CAD build for the part. Positions are in the model's coordinates, mm. A direction names the side the tool comes from. Give positions to 0.01 mm unless a question says otherwise; leave off trailing zeros. Order: outer loops, then holes, each group sorted by start corner. A loop starts at its lowest first (then second) coordinate and runs counter-clockwise, first axis right, second up.
Item 1: Wall check: L1, parallel to Y at x = 4.75, z = 13. Give the ranges that are in metal, low to high.
Item 2: Band-saw the part on C-C on z = 5. Give the cut face in (x, y).
Item 3: Band-saw the part on D-D on x = 4.05. Give the cut face in (y, z), plus the area to 3 significant figures.
Item 4: Which spindle directions (+Z, -Z, +X, -X, +Y, -Y) get a long thin tool onto all of the face, cutting with end or side? Do faces 1 (the flat face through (6.46, -2, 5)), 2 (the cylindrical face through (4.293, -0.986, 0.64)), 3 (the flat face through (0.54, -2, 5)), 4 (the flat face through (1.04, -2, 5)), 5 (the flat face through (5.96, -2, 8)). Say none if no direction does.
Item 5: Band-saw the part on B-B on x = 6.21. Give the cut face in (y, z), plus the area to 3 significant figures.
Item 6: Band-saw the part on A-A on y = -1.5. Give the cut face in (x, z).
Item 7: Two-plate mould, pull along X, no slides. Class faces 6 (the flat face through (4, 7, 13.7)), 7 (the flat face through (0, 7, 7)), 8 (the cylindrical face through (5.84, -0.99, 0.87)): released by +X, released by -X, zero draft, split by the parting line, or undercut.
Item 8: Flat gauge pins, fed straight in: P1, Ø1.2, axis at y = -1.5, z = 5.5, coming from the +X side; P2, Ø5, axis at y = -0.5, z = 3, coming from the +X side; P3, Ø1.6, axis at y = -2, z = 8, coming from the -X side; P4, Ø0.6, axis at x = 4, z = 1, coming from the -Y side. Where does each tip first touch, or does it go through?
```python
from build123d import *

# Parameters (mm, degrees)
ESQUISSE1_W      = 7.25
ESQUISSE1_H      = 14.75
EXTRUSION1_DEPTH = 13.7
EXTRUSION2_DEPTH = 3.65
ESQUISSE3_R      = 0.4
EXTRUSION3_DEPTH = 2


with BuildPart() as part:
    # Esquisse1 → Extrusion1 (new body)
    with BuildSketch(Plane.XY):
        with Locations((3.625, 7.375)):
            Rectangle(ESQUISSE1_W, ESQUISSE1_H)
    extrude(amount=EXTRUSION1_DEPTH)

    # Esquisse2 → Extrusion2 (add)
    with BuildSketch(Plane.XZ):
        with BuildLine():
            Line((1.04, 6.84), (1.04, 8.34))
            ThreePointArc((1.04, 8.34), (0.79, 8.59), (0.54, 8.34))
            Line((0.54, 8.34), (0.54, 6.84))
            ThreePointArc((0.54, 6.84), (0.79, 6.59), (1.04, 6.84))
        make_face()
        with BuildLine():
            Line((6.46, 6.84), (6.46, 8.34))
            ThreePointArc((6.46, 8.34), (6.21, 8.59), (5.96, 8.34))
            Line((5.96, 8.34), (5.96, 6.84))
            ThreePointArc((5.96, 6.84), (6.21, 6.59), (6.46, 6.84))
        make_face()
        with BuildLine():
            Line((1.04, 4.3), (1.04, 5.8))
            ThreePointArc((1.04, 5.8), (0.79, 6.05), (0.54, 5.8))
            Line((0.54, 5.8), (0.54, 4.3))
            ThreePointArc((0.54, 4.3), (0.79, 4.05), (1.04, 4.3))
        make_face()
        with BuildLine():
            Line((5.96, 4.3), (5.96, 5.8))
            ThreePointArc((5.96, 5.8), (6.21, 6.05), (6.46, 5.8))
            Line((6.46, 5.8), (6.46, 4.3))
            ThreePointArc((6.46, 4.3), (6.21, 4.05), (5.96, 4.3))
        make_face()
    extrude(amount=EXTRUSION2_DEPTH)

    # Esquisse3 → Extrusion3 (add)
    with BuildSketch(Plane.XZ):
        with Locations(Location((4.05, 0.956934673, 0), (0, 0, 90))):
            Circle(ESQUISSE3_R)
        with Locations(Location((2.65, 0.956934673, 0), (0, 0, 90))):
            Circle(ESQUISSE3_R)
        with Locations(Location((1.25, 0.956934673, 0), (0, 0, 90))):
            Circle(ESQUISSE3_R)
        with Locations(Location((5.45, 0.956934673, 0), (0, 0, 90))):
            Circle(ESQUISSE3_R)
    extrude(amount=EXTRUSION3_DEPTH)


solid = part.part
```
The answers:
1. L1: y = 0 to 14.75
2. outline: (0, 0) - (0.54, 0) - (0.54, -3.65) - (1.04, -3.65) - (1.04, 0) - (5.96, 0) - (5.96, -3.65) - (6.46, -3.65) - (6.46, 0) - (7.25, 0) - (7.25, 14.75) - (0, 14.75) - close
3. outline: (-2, 0.56) - (0, 0.56) - (0, 0) - (14.75, 0) - (14.75, 13.7) - (0, 13.7) - (0, 1.36) - (-2, 1.36) - close
3. area: 204 mm2
4. face 1: +Z, -Z, +X, -Y
4. face 2: -Y
4. face 3: +Z, -Z, -X, -Y
4. face 4: +Z, -Y
4. face 5: +Z, -Z, -Y
5. outline: (-3.65, 4.05) - (0, 4.05) - (0, 0) - (14.75, 0) - (14.75, 13.7) - (0, 13.7) - (0, 8.59) - (-3.65, 8.59) - (-3.65, 6.59) - (0, 6.59) - (0, 6.05) - (-3.65, 6.05) - close
5. area: 217 mm2
6. outline: (0.54, 4.3) arc R0.25 ccw to (1.04, 4.3) - (1.04, 5.8) arc R0.25 ccw to (0.54, 5.8) - close; (0.54, 6.84) arc R0.25 ccw to (1.04, 6.84) - (1.04, 8.34) arc R0.25 ccw to (0.54, 8.34) - close; circle Ø0.8 at (1.25, 0.96); circle Ø0.8 at (2.65, 0.96); circle Ø0.8 at (4.05, 0.96); circle Ø0.8 at (5.45, 0.96); (5.96, 4.3) arc R0.25 ccw to (6.46, 4.3) - (6.46, 5.8) arc R0.25 ccw to (5.96, 5.8) - close; (5.96, 6.84) arc R0.25 ccw to (6.46, 6.84) - (6.46, 8.34) arc R0.25 ccw to (5.96, 8.34) - close
7. face 6: zero draft
7. face 7: released by -X
7. face 8: undercut
8. P1: stops at x = 6.46
8. P2: stops at x = 7.25
8. P3: stops at x = 0.54
8. P4: stops at y = -2
